```python
from build123d import *

# Parameters (mm, degrees)
SKETCH1_W                      = 25.4
SKETCH1_H                      = 12.6746
BOSS_EXTRUDE1_DEPTH            = 5.159375
SKETCH2_R                      = 2.24917
CUT_EXTRUDE1_DEPTH             = 27.682213583
FILLET1_R                      = 6.35
CBORE_FOR_M2_SHCS1_D           = 2.4
CBORE_FOR_M2_SHCS1_CBORE_D     = 4.4
CBORE_FOR_M2_SHCS1_CBORE_DEPTH = 2


with BuildPart() as part:
    # Sketch1 → Boss-Extrude1 (new body)
    with BuildSketch(Plane.XY):
        with Locations((12.7, 0)):
            Rectangle(SKETCH1_W, SKETCH1_H)
    extrude(amount=BOSS_EXTRUDE1_DEPTH)

    # Sketch2 → Cut-Extrude1 (cut, through all)
    with BuildSketch(Plane.XY.offset(5.159375)):
        with Locations((19.05, 0)):
            Circle(SKETCH2_R)
    extrude(amount=-CUT_EXTRUDE1_DEPTH, mode=Mode.SUBTRACT)

    # Fillet1
    # the kernel refuses this fillet: 6.35 mm, written as the material it takes off along each edge
    with BuildSketch(Plane(origin=(25.4, -6.3373, -15.875), x_dir=(0, 1, 0), z_dir=(0, 0, 1)), Plane(origin=(25.4, 6.3373, -15.875), x_dir=(-1, 0, 0), z_dir=(0, 0, 1))) as fillet1_piece_1:
        with BuildLine():
            CenterArc((FILLET1_R, FILLET1_R), FILLET1_R, 180, 90)
            Line((0, FILLET1_R), (0, 0))
            Line((0, 0), (FILLET1_R, 0))
        make_face()
    extrude(amount=36.909375, mode=Mode.SUBTRACT)

    # CBORE for M2 SHCS1 (through all)
    with Locations(Plane.XY.offset(5.159375)):
        with Locations((2.38125, 3.96875), (2.38125, -3.96875)):
            CounterBoreHole(CBORE_FOR_M2_SHCS1_D / 2, CBORE_FOR_M2_SHCS1_CBORE_D / 2, CBORE_FOR_M2_SHCS1_CBORE_DEPTH)


solid = part.part
```
Model file for the job. Use its own axes, mm. A direction names the side the tool comes from. Coordinates: 2 decimals unless noted, no trailing zeros. Write each loop counter-clockwise with the first axis right and the second up, starting at its lowest first coordinate (ties: lowest second). Pieces come first, ordered by that corner, then holes. Notation, with made-up numbers: (77, 15.5) - (100, 15.5) arc R23 ccw to (100, 25.5) - close; hole circle Ø5 at (11, -10). An arc over 180 degrees is marked (long way). One line per item, written item: value. Start each with the question number.
1. Probe line 1 (Y direction, x = 3.5, z = 3.55); line 2 (X direction, y = -0.5, z = 4.2); line 3 (X direction, y = -3.75, z = 0.35). List the from-to ranges inside material, lowest first. Write a range as from..to.
2. Slice it at A-A (y = 4.25). Write the cut outline in (x, z).
3. Tool access for faces 5 (the cylindrical face through (1.736, 4.981, 1.558)), 6 (the flat face through (2.4, -5.4, 3.159)): list every direction of +Z, -Z, +X, -X, +Y, -Y with a clear straight run to the whole face (end or side of a thin tool).
4. Flat gauge pins, fed straight in: pin 1 (1 mm diameter, centred on y = -4, z = 1, fed in from +X); pin 2 (3 mm diameter, centred on x = 2.38, y = 3.97, fed in from +Z); pin 3 (1.3 mm diameter, centred on x = 2, y = -4, fed in from +Z). Where does each tip first touch, or does it go through?
5. Slice it at C-C (z = 0.9). Write the cut outline in (x, y), plus the area to 3 significant figures.
6. Mould opens along Y. For faces 1 (the flat face through (0, 0, 3)), 2 (the flat face through (9, 6.337, 3)), 3 (the flat face through (9, -6.337, 3)), 4 (the cylindrical face through (0.635, 2.63, 4.173)) say: released by +Y, released by -Y, zero draft, split by the parting line, or undercut.
7. Slice it at D-D (y = -3.25). Write the cut outline in (x, z).
8. Slice it at B-B (x = 20). Write the cut outline in (y, z), plus the area to 3 significant figures.
Answers below:
1. line 1: y = -6.34..-5.86, -2.07..2.07, 5.86..6.34
1. line 2: x = 0..16.86, 21.24..25.38
1. line 3: x = 0..1.2, 3.56..24.17
2. outline: (0, 0) - (1.21, 0) - (1.21, 3.16) - (0.2, 3.16) - (0.2, 5.16) - (0, 5.16) - close; (3.55, 0) - (23.76, 0) - (23.76, 5.16) - (4.56, 5.16) - (4.56, 3.16) - (3.55, 3.16) - close
3. face 5: +Z, -Z
3. face 6: +Z
4. pin 1: stops at x = 24.34
4. pin 2: stops at z = 3.16
4. pin 3: passes through
5. outline: (0, -6.34) - (19.05, -6.34) arc R6.35 ccw to (25.4, 0) arc R6.35 ccw to (19.05, 6.34) - (0, 6.34) - close; hole circle Ø2.4 at (2.38, -3.97); hole circle Ø2.4 at (2.38, 3.97); hole circle Ø4.5 at (19.05, 0)
5. area: 280 mm^2
6. face 1: zero draft
6. face 2: released by +Y
6. face 3: released by -Y
6. face 4: undercut
7. outline: (0, 0) - (1.42, 0) - (1.42, 3.16) - (0.3, 3.16) - (0.3, 5.16) - (0, 5.16) - close; (3.34, 0) - (24.5, 0) - (24.5, 5.16) - (4.46, 5.16) - (4.46, 3.16) - (3.34, 3.16) - close
8. outline: (-6.27, 0) - (-2.04, 0) - (-2.04, 5.16) - (-6.27, 5.16) - close; (2.04, 0) - (6.27, 0) - (6.27, 5.16) - (2.04, 5.16) - close
8. area: 43.6 mm^2
